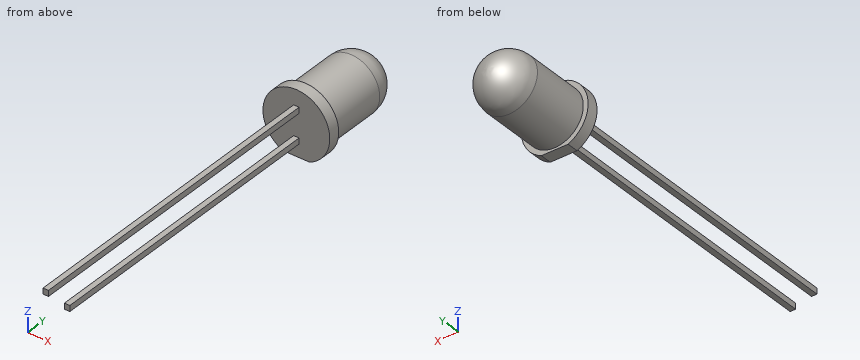
from build123d import *

# Parameters (mm, degrees)
EXTRUDE_1_DEPTH = 1
SKETCH_2_R      = 2.46
EXTRUDE_2_DEPTH = 7.6
SKETCH_4_W      = 0.47
SKETCH_4_H      = 0.5
EXTRUDE_3_DEPTH = 25.7
SKETCH_5_W      = 0.47
SKETCH_5_H      = 0.5
EXTRUDE_4_DEPTH = 2.4


with BuildPart() as part:
    # 草图1 → 凸台-拉伸1 (new body)
    with BuildSketch(Plane(origin=(0, 0, 0), x_dir=(1, 0, 0), z_dir=(0, 1, 0))):
        with BuildLine():
            Line((-1.149957, 2.635), (1.149957, 2.635))
            ThreePointArc((1.149957, 2.635), (0, -2.875), (-1.149957, 2.635))
        make_face()
    extrude(amount=EXTRUDE_1_DEPTH)

    # 草图2 → 凸台-拉伸2 (add)
    with BuildSketch(Plane(origin=(0, 1, 0), x_dir=(1, 0, 0), z_dir=(0, 1, 0))):
        Circle(SKETCH_2_R)
    extrude(amount=EXTRUDE_2_DEPTH)

    # 草图3 → 切除-旋转1 (revolve, cut)
    with BuildSketch(Plane(origin=(0, 0, 0), x_dir=(0, 0, -1), z_dir=(1, 0, 0))):
        with BuildLine():
            Line((-2.46, 6.14), (-4.608425, 6.14))
            Line((-4.608425, 6.14), (-4.608425, 10.205518))
            Line((-4.608425, 10.205518), (0, 10.205518))
            Line((0, 10.205518), (0, 8.6))
            ThreePointArc((0, 8.6), (-1.739483, 7.879483), (-2.46, 6.14))
        make_face()
    revolve(axis=Axis((0, 10.969013, 0), (0, -1, 0)), mode=Mode.SUBTRACT)

    # 草图4 → 凸台-拉伸3 (add)
    with BuildSketch(Plane.XZ):
        with Locations((0, -1.265)):
            Rectangle(SKETCH_4_W, SKETCH_4_H)
        with Locations((0, 1.265)):
            Rectangle(SKETCH_4_W, SKETCH_4_H)
    extrude(amount=EXTRUDE_3_DEPTH)

    # 草图5 → 凸台-拉伸4 (add)
    with BuildSketch(Plane.XZ.offset(25.7)):
        with Locations((0, 1.265)):
            Rectangle(SKETCH_5_W, SKETCH_5_H)
    extrude(amount=EXTRUDE_4_DEPTH)


solid = part.part
Work out the finished part from the listing and answer in its coordinate system (mm). Give positions to 0.01 mm unless a question says otherwise; leave off trailing zeros. Order: outer loops, then holes, each group sorted by start corner. A loop starts at its lowest first (then second) coordinate and runs counter-clockwise, first axis right, second up. Notation, with made-up numbers: (69.25, 41) - (90.25, 41) arc R7 cw to (90.25, 46) - close; hole circle Ø6 at (32.25, 39). An arc over 180 degrees is marked (long way). Answer as CSV lines item,"result". Start each with the question number.
Q1. The part is cut by section B-B (y = 4.5). Write down the section's boundary in (x, z).
Q2. The part is cut by section A-A (y = -0.5). Write down the section's boundary in (x, z) (3 decimals).
Q3. Find the intervals of material crossed by L1, parallel to Z at x = 0.15, y = -6.5 (3 decimals); L2, parallel to Y at x = 2.45, z = -1.3; L3, parallel to X at y = -23, z = -1.4 (3 decimals), in increasing order. Write a range as [from, to].
Q4. Given pin 1 Ø0.6 at (y, z) = (-9, -1) entering from +X (3 decimals); pin 2 Ø0.6 at (y, z) = (-11.5, -1) entering from -X (3 decimals); pin 3 Ø0.5 at (x, z) = (0, -1) entering from -Y, each flat-ended and moving along its own axis, determine where each tip first touches the part or whether it passes through.
Check result:
1,outline,"circle Ø4.92 at (0, 0)"
2,outline,"(-0.235, -1.515) - (0.235, -1.515) - (0.235, -1.015) - (-0.235, -1.015) - close; (-0.235, 1.015) - (0.235, 1.015) - (0.235, 1.515) - (-0.235, 1.515) - close"
3,L1,"z = [-1.515, -1.015], [1.015, 1.515]"
3,L2,"y = [0, 1]"
3,L3,"x = [-0.235, 0.235]"
4,pin 1,"stops at x = 0.235"
4,pin 2,"stops at x = -0.235"
4,pin 3,"stops at y = -25.7"
